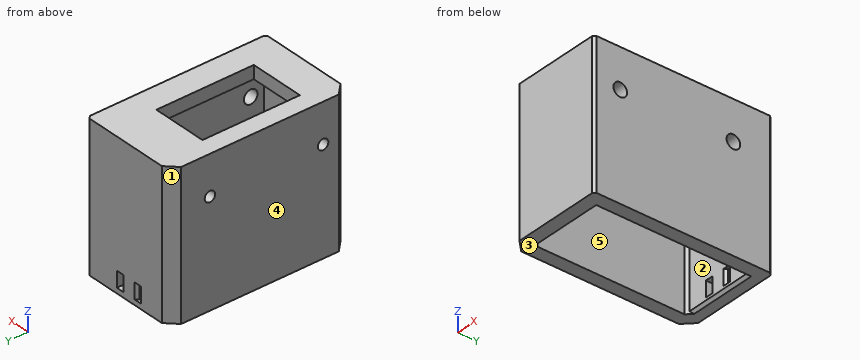
Autodesk Fusion 360 part; units mm, degrees
sketch "Sketch1" plane through (0, 0, 0) normal (0, 0, 1) x (1, 0, 0)
  line L0 (10.5, -18.575) -> (-10.5, -18.575)
  line L1 (-10.5, -18.575) -> (-10.5, 18.575)
  line L2 (-10.5, 18.575) -> (10.5, 18.575)
  line L3 (10.5, 18.575) -> (10.5, -18.575)
  line L4 (10.5, -18.575) -> (-10.5, 18.575) construction
  line L5 (-10.5, -18.575) -> (10.5, 18.575) construction
  line L6 (15.5, -26.575) -> (-12.5, -26.575)
  line L7 (-12.5, -26.575) -> (-12.5, 31.575)
  line L8 (-12.5, 31.575) -> (15.5, 31.575)
  line L9 (15.5, 31.575) -> (15.5, -26.575)
  line L10 (20.5, -31.575) -> (-17.5, -31.575)
  line L11 (-17.5, -31.575) -> (-17.5, 36.575)
  line L12 (-17.5, 36.575) -> (20.5, 36.575)
  line L13 (20.5, 36.575) -> (20.5, -31.575)
  dimension "d1" = 21
  dimension "d2" = 37.15
  dimension "d4" = 2
  dimension "d5" = 8
  dimension "d6" = 5
  dimension "d7" = 5
  dimension "d19" = 13
  dimension "d20" = 5
  dimension "d21" = 5
  dimension "d22" = 5
extrude "Extrude1" add sketch "Sketch1" against normal blind 5 contours L6 L7 L8 L9
extrude "Extrude2" add sketch "Sketch1" against normal blind 55 contours L10 L11 L12 L13
sketch "Sketch3" plane through (20.5, 0, 0) normal (1, 0, 0) x (0, 1, 0)
  line L0 (36.575, 0) -> (-31.575, 0)
  line L1 (-31.575, 0) -> (-31.575, -55)
  line L2 (-31.575, -55) -> (36.575, -55)
  line L3 (36.575, -55) -> (36.575, 0)
  line L4 (-31.575, -15) -> (36.575, -15) construction
  line L5 (36.575, 0) -> (-31.575, 0)
  circle A0 centre (21.575, -15) radius 2.6
  circle A1 centre (-21.575, -15) radius 2.6
  line L6 (-26.575, -5) -> (31.575, -5)
  line L7 (31.575, -5) -> (31.575, -55)
  line L8 (31.575, -55) -> (-26.575, -55)
  line L9 (-26.575, -55) -> (-26.575, -5)
  dimension "d23" = 15
  dimension "d24" = 5.2
  dimension "d25" = 5.2
  dimension "d26" = 10
  dimension "d27" = 5
extrude "Extrude4" cut sketch "Sketch3" against normal up to surface (5 mm away) contours A0 | A1
sketch "Sketch4" plane through (-17.5, 0, 0) normal (-1, 0, 0) x (0, -1, 0)
  line L0 (31.575, 0) -> (-36.575, 0)
  line L1 (-36.575, 0) -> (-36.575, -55)
  line L2 (-36.575, -55) -> (31.575, -55)
  line L3 (31.575, -55) -> (31.575, 0)
  circle A0 centre (21.575, -15) radius 2.6
  circle A1 centre (-21.575, -15) radius 2.6
  line L4 (26.575, -5) -> (-31.575, -5)
  line L5 (-31.575, -5) -> (-31.575, -55)
  line L6 (-31.575, -55) -> (26.575, -55)
  line L7 (26.575, -55) -> (26.575, -5)
  circle A2 centre (-21.575, -15) radius 2
  circle A3 centre (21.575, -15) radius 2
  dimension "d30" = 4
  dimension "d31" = 4
chamfer "Chamfer5" distance 1 angle 45 2 edges at (-12.5, -26.575, -30) (-12.5, 31.575, -30)
extrude "Extrude5" cut sketch "Sketch4" against normal through all contours A2 | A3
sketch "Sketch5" plane through (0, 36.575, 0) normal (0, 1, 0) x (-1, 0, 0)
  line L0 (-20.5, -55) -> (17.5, -55)
  line L1 (17.5, 0) -> (-20.5, 0)
  line L2 (-1.5, -55) -> (-1.5, 0) construction
  line L3 (2, -47) -> (4, -47)
  line L4 (4, -47) -> (4, -53)
  line L5 (4, -53) -> (2, -53)
  line L6 (2, -53) -> (2, -47)
  line L7 (-7, -47) -> (-7, -53)
  line L8 (-7, -53) -> (-5, -53)
  line L9 (-5, -53) -> (-5, -47)
  line L10 (-5, -47) -> (-7, -47)
  line L11 (17.5, -55) -> (17.5, 0)
  line L12 (-20.5, 0) -> (-20.5, -55)
  dimension "d35" = 6
  dimension "d36" = 2
  dimension "d37" = 3.5
  dimension "d38" = 2
extrude "Extrude6" cut sketch "Sketch5" against normal up to surface (5 mm away) contours L3 L4 L5 L6 | L7 L8 L9 L10
chamfer "Chamfer2" distance 1 angle 45 2 edges at (5, 31.575, -50) (-2, 31.575, -50)
chamfer "Chamfer3" distance 1 angle 45 2 edges at (5, 36.575, -50) (-2, 36.575, -50)
chamfer "Chamfer4" distance 1 angle 45 1 edges at (1.5, 31.575, -55)
chamfer "Chamfer1" distance 1 angle 45 2 edges at (20.5, 36.575, -27.5) (20.5, -31.575, -27.5)
chamfer "Chamfer6" distance 4 angle 45 2 edges at (-17.5, 36.575, -27.5) (-17.5, -31.575, -27.5)
equation "d30 = d31"
Could you check a few things on this model? Use its own coordinates, in mm. Face numbers are marked on the shaded views. A direction names the side the tool comes from. Give positions to 0.01 mm unless a question says otherwise; leave off trailing zeros. Order: outer loops, then holes, each group sorted by start corner. A loop starts at its lowest first (then second) coordinate and runs counter-clockwise, first axis right, second up.
1. Suppose I cut it at C-C (x = 8.5). List the corners of the cut face in (y, z) for me (3 decimals), plus the area to 4 significant figures.
2. Suppose I cut it at A-A (y = 9). List the corners of the cut face in (x, z) for me.
3. Will these pins go through, and if not, where does the flat tip stop? P1, Ø10, axis at x = 9, y = 8, coming from the -Z side; P2, Ø1.5, axis at y = 34, z = -48.5, coming from the -X side (3 decimals); P3, Ø4.5, axis at y = -21.575, z = -15, coming from the +X side.
4. I need wall thicknesses on L1, parallel to Y at x = 0, z = -12 (3 decimals); L2, parallel to X at y = -10.5, z = -38; L3, parallel to Z at x = 6.5, y = 33. Which ranges of each line are inside material? Lowest first, please.
5. For the marked faces 1 and 2, which set-ups out of +Z, -Z, +X, -X, +Y, -Y let a thin tool reach every point of the face, with its end or its side?
6. We'd pull the mould along X, two halves only. Please class the marked faces 3, 4 and 5: pulls with the +X half, pulls with the -X half, needs draft (parallel to the pull), parting line crosses it, or undercut.
7. Suppose I cut it at D-D (z = -33). List the corners of the cut face in (x, y) for me (3 decimals), plus the area to 4 significant figures.
8. Suppose I cut it at B-B (z = -15). Give the number of separate pieces and of enclosed holes in the cut face, plus the area to 4 significant figures.
Solved:
1. outline: (-31.575, -55) - (-26.575, -55) - (-26.575, -5) - (-18.575, -5) - (-18.575, 0) - (-31.575, 0) - close; (18.575, -5) - (31.575, -5) - (31.575, -54) - (32.575, -55) - (36.575, -55) - (36.575, 0) - (18.575, 0) - close
1. area: 654.5 mm2
2. outline: (-17.5, -55) - (-12.5, -55) - (-12.5, -5) - (-10.5, -5) - (-10.5, 0) - (-17.5, 0) - close; (10.5, -5) - (15.5, -5) - (15.5, -55) - (20.5, -55) - (20.5, 0) - (10.5, 0) - close
3. P1: stops at z = -5
3. P2: stops at x = -16.825
3. P3: stops at x = -12.5
4. L1: y = -31.575 to -26.575, 31.575 to 36.575
4. L2: x = -17.5 to -12.5, 15.5 to 20.5
4. L3: z = -55 to -53, -47 to 0
5. face 1: +Z, -Z, -X, +Y
5. face 2: -Z
6. face 3: needs draft
6. face 4: pulls with the -X half
6. face 5: undercut
7. outline: (-17.5, -27.575) - (-13.5, -31.575) - (19.5, -31.575) - (20.5, -30.575) - (20.5, 35.575) - (19.5, 36.575) - (-13.5, 36.575) - (-17.5, 32.575) - close; hole (-12.5, -25.575) - (-11.5, -26.575) - (15.5, -26.575) - (15.5, 31.575) - (-11.5, 31.575) - (-12.5, 30.575) - close
7. area: 945.5 mm2
8. separate pieces: 4
8. enclosed holes: 0
8. area: 853.5 mm2
